The listing builds one solid part. Answer for the finished solid, in the listing's coordinates (mm). A direction names the side the tool comes from. Coordinates: 2 decimals unless noted, no trailing zeros. Write each loop counter-clockwise with the first axis right and the second up, starting at its lowest first coordinate (ties: lowest second). Pieces come first, ordered by that corner, then holes.
Autodesk Inventor part; units mm, degrees
ref_plane "YZ Plane" through (0, 0, 0) normal (1, 0, 0) x (0, 1, 0)
ref_plane "XZ Plane" through (0, 0, 0) normal (0, 1, 0) x (-1, 0, 0)
ref_plane "XY Plane" through (0, 0, 0) normal (0, 0, 1) x (1, 0, 0)
sketch "スケッチ1" plane through (0, 0, 0) normal (0, 0, 1) x (1, 0, 0)
  line L0 (0, 0) -> (10, 0)
  line L1 (10, 0) -> (10, 1.5)
  line L2 (10, 1.5) -> (0, 1.5)
  line L3 (0, 1.5) -> (0, 0)
  line L4 (0, 0) -> (0, 2.75)
  line L5 (0, 0) -> (-2, 0)
  line L6 (-2, 0) -> (0, 0)
  line L7 (-2, 0) -> (-2, 1.15)
  line L8 (0, 0) -> (-2, 0)
  line L9 (-2, 0) -> (-2, 2.75)
  line L10 (-2, 2.75) -> (0, 2.75)
  line L11 (0, 2.75) -> (0, 0)
  dimension "d0" = 1.5
  dimension "d1" = 10
  dimension "d3" = 2
  dimension "d4" = 2.75
  dimension "d5" = 1.15
revolve "回転1" add sketch "スケッチ1" angle 360 about axis through (-2, 0, 0) along (1, 0, 0)
thread "ねじ1"
sketch "スケッチ2" plane through (-2, 0, 0) normal (-1, 0, 0) x (0, 0, 1)
  circle A0 centre (0, 0) radius 1.15
  line L0 (-0.575, 0.9959) -> (0.575, 0.9959)
  line L1 (0.575, 0.9959) -> (1.15, 0)
  line L2 (1.15, 0) -> (0.575, -0.9959)
  line L3 (0.575, -0.9959) -> (-0.575, -0.9959)
  line L4 (-0.575, -0.9959) -> (-1.15, 0)
  line L5 (-1.15, 0) -> (-0.575, 0.9959)
  dimension "d10" = 1.15
  dimension "d11" = 1.9919
extrude "押し出し1" cut sketch "スケッチ2" against normal blind 1.4 contours L2 L3 L4 L5 L0 L1
fillet "フィレット1" radius 0.2 6 edges at (-0.6, 0.9959, 0) (-0.6, 0.498, 0.8625) (-0.6, 0.498, -0.8625) (-0.6, -0.498, -0.8625) (-0.6, -0.9959, 0) (-0.6, -0.498, 0.8625)
fillet "フィレット2" radius 0.1 1 edges at (0, -1.5, 0)
fillet "フィレット3" radius 0.1 1 edges at (10, -1.5, 0)
properties part number "ネジキャップM3L10" material "鋼"
Q1. Find the intervals of material crossed by probe 1 along X at (y, z) = (1.6, 0.3); probe 2 along Z at (x, y) = (1.5, -1.15); probe 3 along Z at (x, y) = (0.75, -0.5), in increasing order.
Answers below:
probe 1: x = -2 to 0
probe 2: z = -0.96 to 0.96
probe 3: z = -1.41 to 1.41
Q2. The part is cut by section B-B, the plane z = 0. Write down the section's boundary in (x, y), then the cut area to 3 significant figures.
Answers below:
outline: (-2, -2.75) - (0, -2.75) - (0, -1.6) arc R0.1 cw to (0.1, -1.5) - (9.9, -1.5) arc R0.1 ccw to (10, -1.4) - (10, 1.4) arc R0.1 ccw to (9.9, 1.5) - (0.1, 1.5) arc R0.1 cw to (0, 1.6) - (0, 2.75) - (-2, 2.75) - (-2, 1) - (-0.8, 1) arc R0.2 cw to (-0.6, 0.8) - (-0.6, -0.8) arc R0.2 cw to (-0.8, -1) - (-2, -1) - close
area: 38.2 mm2
Q3. The part is cut by section C-C, the plane x = 8.5. Write down the section's boundary in (y, z).
Answers below:
outline: circle Ø3 at (0, 0)
Q4. Given pin 1 (2 mm diameter, centred on x = 6.5, y = 1.5, fed in from +Z); pin 2 (1.5 mm diameter, centred on x = 2, y = -1, fed in from +Z); pin 3 (3 mm diameter, centred on x = 8.5, z = 0.5, fed in from +Y), each flat-ended and moving along its own axis, determine where each tip first touches the part or whether it passes through.
Answers below:
pin 1: stops at z = 1.41
pin 2: stops at z = 1.48
pin 3: stops at y = 1.5
Q5. Which of the six approach directions +Z, -Z, +X, -X, +Y, -Y give full straight-line access (tool end or side, diameter ignored) to faces 4 (the face through (-0.6, 0, 0)), 5 (the face through (0, 2, 0)), 6 (the face through (10, 0, 0))?
Answers below:
face 4: -X
face 5: +X
face 6: +Z, -Z, +X, +Y, -Y
Q6. The part is cut by section D-D, the plane z = -2.35. Write down the section's boundary in (x, y), then the cut area to 3 significant figures.
Answers below:
outline: (-2, -1.43) - (0, -1.43) - (0, 1.43) - (-2, 1.43) - close
area: 5.71 mm2
Q7. The part is cut by section A-A, the plane x = -1. Write down the section's boundary in (y, z) (3 decimals).
Answers below:
outline: circle Ø5.5 at (0, 0); hole (-0.996, -0.575) - (0, -1.15) - (0.996, -0.575) - (0.996, 0.575) - (0, 1.15) - (-0.996, 0.575) - close
Q8. Determine the mould class of faces 1 (the face through (4.93, -1.5, -0.07)), 2 (the face through (-2, 1.2, 0)), 3 (the face through (-1, -0.996, 0)) for opening direction Z: released by +Z, released by -Z, zero draft, split by the parting line, or undercut.
Answers below:
face 1: split by the parting line
face 2: zero draft
face 3: undercut
